Autodesk Inventor part; units mm, degrees
ref_plane "YZ Plane" through (0, 0, 0) normal (1, 0, 0) x (0, 1, 0)
ref_plane "XZ Plane" through (0, 0, 0) normal (0, 1, 0) x (-1, 0, 0)
ref_plane "XY Plane" through (0, 0, 0) normal (0, 0, 1) x (1, 0, 0)
sketch "スケッチ1" plane through (-150, -150, 0) normal (0, 0, 1) x (1, 0, 0)
  circle A0 centre (59.9853, 240.0147) radius 24 construction
  circle A1 centre (59.9853, 240.0147) radius 24 construction
  circle A2 centre (84.0269, 264.0563) radius 10 construction
  line L0 (84.0269, 264.0563) -> (59.9853, 240.0147) construction
  line L1 (59.9853, 240.0147) -> (84.0269, 215.9731) construction
  arc A3 (84.5273, 253.0677) -> (73.0383, 264.5567) centre (84.0269, 264.0563) ccw
  arc A4 (70.2215, 262.823) -> (82.7936, 250.2509) centre (59.9853, 240.0147) ccw
  arc A5 (84.5273, 253.0677) -> (82.7936, 250.2509) centre (84.6183, 251.0698) ccw
  arc A6 (70.2215, 262.823) -> (73.0383, 264.5567) centre (71.0404, 264.6477) ccw
  line L2 (67.0564, 275.37) -> (24.63, 232.9436) construction
  line L3 (24.63, 232.9436) -> (52.9142, 204.6594) construction
  line L4 (52.9142, 204.6594) -> (95.3406, 247.0858) construction
  line L5 (95.3406, 247.0858) -> (67.0564, 275.37) construction
  line L6 (67.0564, 275.37) -> (52.9142, 204.6594) construction
  line L7 (24.63, 232.9436) -> (95.3406, 247.0858) construction
  circle A7 centre (95.3406, 247.0858) radius 1.6
  circle A8 centre (52.9142, 204.6594) radius 1.6
  circle A9 centre (24.63, 232.9436) radius 1.6
  circle A10 centre (67.0564, 275.37) radius 1.6
  line L8 (270, 30) -> (30, 30) construction
  line L9 (30, 30) -> (30, 270) construction
  line L10 (30, 270) -> (270, 270) construction
  line L11 (270, 270) -> (270, 30) construction
  line L12 (270, 30) -> (30, 270) construction
  line L13 (30, 30) -> (270, 270) construction
  circle A11 centre (30, 270) radius 2 construction
  circle A12 centre (270, 270) radius 2 construction
  circle A13 centre (30, 30) radius 2
  circle A14 centre (270, 30) radius 2
  circle A15 centre (150, 150) radius 30
  line L14 (150, 113) -> (117.9571, 131.5) construction
  line L15 (117.9571, 131.5) -> (117.9571, 168.5) construction
  line L16 (117.9571, 168.5) -> (150, 187) construction
  line L17 (150, 187) -> (182.0429, 168.5) construction
  line L18 (182.0429, 168.5) -> (182.0429, 131.5) construction
  line L19 (182.0429, 131.5) -> (150, 113) construction
  circle A16 centre (150, 150) radius 37 construction
  circle A17 centre (150, 113) radius 1.6
  circle A18 centre (54.1207, 93.2509) radius 1.6 construction
  line L20 (117.9571, 131.5) -> (117.9571, 168.5) construction
  line L21 (150, 113) -> (117.9571, 131.5) construction
  line L22 (117.9571, 168.5) -> (150, 187) construction
  line L23 (182.0429, 131.5) -> (150, 113) construction
  circle A19 centre (150, 150) radius 30 construction
  line L24 (150, 187) -> (182.0429, 168.5) construction
  line L25 (182.0429, 168.5) -> (182.0429, 131.5) construction
  circle A20 centre (150, 150) radius 37 construction
  circle A21 centre (182.0429, 131.5) radius 1.6
  circle A22 centre (151.2065, 38.5916) radius 1.6 construction
  line L26 (150, 113) -> (117.9571, 131.5) construction
  line L27 (182.0429, 131.5) -> (150, 113) construction
  line L28 (117.9571, 131.5) -> (117.9571, 168.5) construction
  line L29 (182.0429, 168.5) -> (182.0429, 131.5) construction
  circle A23 centre (150, 150) radius 30 construction
  line L30 (117.9571, 168.5) -> (150, 187) construction
  line L31 (150, 187) -> (182.0429, 168.5) construction
  circle A24 centre (150, 150) radius 37 construction
  circle A25 centre (182.0429, 168.5) radius 1.6
  circle A26 centre (247.0858, 95.3406) radius 1.6 construction
  line L32 (182.0429, 131.5) -> (150, 113) construction
  line L33 (182.0429, 168.5) -> (182.0429, 131.5) construction
  line L34 (150, 113) -> (117.9571, 131.5) construction
  line L35 (150, 187) -> (182.0429, 168.5) construction
  circle A27 centre (150, 150) radius 30 construction
  line L36 (117.9571, 131.5) -> (117.9571, 168.5) construction
  line L37 (117.9571, 168.5) -> (150, 187) construction
  circle A28 centre (150, 150) radius 37 construction
  circle A29 centre (150, 187) radius 1.6
  circle A30 centre (245.8793, 206.7491) radius 1.6 construction
  line L38 (182.0429, 168.5) -> (182.0429, 131.5) construction
  line L39 (150, 187) -> (182.0429, 168.5) construction
  line L40 (182.0429, 131.5) -> (150, 113) construction
  line L41 (117.9571, 168.5) -> (150, 187) construction
  circle A31 centre (150, 150) radius 30 construction
  line L42 (150, 113) -> (117.9571, 131.5) construction
  line L43 (117.9571, 131.5) -> (117.9571, 168.5) construction
  circle A32 centre (150, 150) radius 37 construction
  circle A33 centre (117.9571, 168.5) radius 1.6
  circle A34 centre (148.7935, 261.4084) radius 1.6 construction
  line L44 (150, 187) -> (182.0429, 168.5) construction
  line L45 (117.9571, 168.5) -> (150, 187) construction
  line L46 (182.0429, 168.5) -> (182.0429, 131.5) construction
  line L47 (117.9571, 131.5) -> (117.9571, 168.5) construction
  circle A35 centre (150, 150) radius 30 construction
  line L48 (182.0429, 131.5) -> (150, 113) construction
  line L49 (150, 113) -> (117.9571, 131.5) construction
  circle A36 centre (150, 150) radius 37 construction
  circle A37 centre (117.9571, 131.5) radius 1.6
  line L50 (0, 300) -> (300, 300)
  line L51 (300, 300) -> (300, 0)
  line L52 (300, 0) -> (0, 0)
  line L53 (0, 0) -> (0, 300)
  line L54 (0, 300) -> (300, 0) construction
  line L55 (300, 300) -> (0, 0) construction
  point P0 (150, 150)
  point P1 (81.1985, 261.2279)
  point P2 (150, 150)
  point P3 (59.8791, 125.8522)
  point P4 (150, 150)
  point P5 (125.8522, 59.8791)
  point P6 (150, 150)
  point P7 (215.9731, 84.0269)
  point P8 (150, 150)
  point P9 (240.1209, 174.1478)
  point P10 (150, 150)
  point P11 (174.1478, 240.1209)
  dimension "d30" = 74
  dimension "d6" = 48
  dimension "d7" = 20
  dimension "d10" = 25
  dimension "d11" = 11
  dimension "d12" = 2
  dimension "d15" = 40
  dimension "d16" = 60
  dimension "d17" = 3.2
  dimension "d18" = 240
  dimension "d19" = 4
  dimension "d22" = 240
  dimension "d25" = 240
  dimension "d28" = 60
  dimension "d31" = 3.2
  dimension "d34" = 360
  dimension "d36" = 300
  dimension "d39" = 127.3
  dimension "d40" = 3.2
  dimension "d41" = 48
extrude "押し出し2" add sketch "スケッチ1" along normal blind 10
sketch "スケッチ2" plane through (-150, -150, 0) normal (0, 0, -1) x (-1, 0, 0)
  circle A0 centre (-150, 150) radius 90
  dimension "d42" = 180
extrude "押し出し3" cut sketch "スケッチ2" against normal blind 3
sketch "スケッチ3" plane through (-150, -150, 10) normal (0, 0, 1) x (1, 0, 0)
  line L0 (300, 300) -> (0, 300)
  line L1 (0, 300) -> (0, 0)
  line L2 (0, 0) -> (300, 0)
  line L3 (300, 0) -> (300, 300)
  circle A0 centre (150, 150) radius 30
  line L4 (150, 180) -> (150, 150) construction
  line L5 (50, 180) -> (50, 150)
  line L6 (250, 150) -> (250, 180)
  arc A1 (250, 180) -> (50, 180) centre (150, 180) ccw
  arc A2 (50, 150) -> (250, 150) centre (150, 150) ccw
  line L7 (50, 180) -> (0, 180)
  line L8 (250, 180) -> (300, 180)
  line L9 (300, 40) -> (0, 40)
  line L10 (64, 300) -> (34, 270)
  line L11 (266, 270) -> (236, 300)
  line L12 (300, 270) -> (266, 270)
  line L13 (34, 270) -> (0, 270)
  point P0 (150, 165)
  dimension "d45" = 100
  dimension "d46" = 30
  dimension "d51" = 40
  dimension "d52" = 45
  dimension "d53" = 64
  dimension "d55" = 30
extrude "押し出し5" cut sketch "スケッチ3" against normal blind 10 contours L3 L12 L11 L0 | L10 L13 L1 L0 | L3 L9 L1 L7 L5 A2 L6 L8 | L3 L2 L1 L9
sketch "スケッチ5" plane through (-150, -150, 10) normal (0, 0, 1) x (1, 0, 0)
  circle A0 centre (18, 187) radius 1.6
  circle A1 centre (282, 187) radius 1.6
  point P0 (150, 150)
  point P1 (18, 220)
  point P2 (282, 220)
  dimension "d65" = 33
  dimension "d66" = 33
hole "穴1" at (-132, 37, 10) at (132, 37, 10) at (132, 70, 10) at (-132, 70, 10) direction (0, 0, -1) diameter 3.2 end through all
fillet "フィレット1" radius 3 10 edges at (-86, 150, 5) (-116, 120, 5) (-150, 120, 5) (-150, 30, 5) (-100, 30, 5) (100, 30, 5) (150, 30, 5) (150, 120, 5) (116, 120, 5) (86, 150, 5)
properties part number "ロボットベース2019" material "マツ材"
Input: part model. Units: mm. Frame: model coordinates. A direction names the side the tool comes from. Give positions to 0.01 mm unless a question says otherwise; leave off trailing zeros. Write each loop counter-clockwise with the first axis right and the second up, starting at its lowest first coordinate (ties: lowest second). Pieces come first, ordered by that corner, then holes. Notation, with made-up numbers: M -3,22 L 36,22 A20 ccw 36,33 Z; hole C 12,-12 d4. An arc over 180 degrees is marked long. Use one line per item in the form item = value.
1. First-contact query: P1, Ø4, axis at x = -32.04, y = -18.5, coming from the -Z side; P2, Ø5, axis at x = -121.5, z = 6.5, coming from the -Y side; P3, Ø3, axis at x = -97.09, y = 54.66, coming from the +Z side; P4, Ø3, axis at x = 134, z = 5, coming from the +Y side. Flat tips, straight axial feed; report the tip coordinate or a pass-through.
Outcome:
P1 = 3
P2 = 30
P3 = through
P4 = 120
2. Cut plane A-A on y = -48. Return loops of the section in (x, z).
Outcome:
outline = M -87.73,0 L -76.13,0 L -76.13,3 L 76.13,3 L 76.13,0 L 87.73,0 L 87.73,10 L -87.73,10 Z
3. Cut plane C-C on z = 6. State how many separate pieces and enclosed holes the cut face has, and give its area (3 significant figures).
Outcome:
separate_pieces = 1
enclosed_holes = 16
area = 49,500 mm²
4. Mould query, pull axis X, two halves, no side actions, for faces 1 (the face through (-0.7, 90.4, 0)), 2 (the face through (-2.199, -99.976, 5.07)), 3 (the face through (-106.99, 71.66, 4.93)). Classes: released by +X, released by -X, zero draft, split by the parting line, or undercut.
Outcome:
face_1 = zero draft
face_2 = split by the parting line
face_3 = undercut
5. Ray query, L1, parallel to Y at x = -132, z = 7.5; L2, parallel to Y at x = 0, z = 8.25; L3, parallel to X at y = 37, z = 5.75. Return the intervals inside material, ascending.
Outcome:
L1 = 30 to 35.4, 38.6 to 68.4, 71.6 to 120
L2 = -100 to -38.6, -35.4 to -30, 30 to 35.4, 38.6 to 150
L3 = -150 to -133.6, -130.4 to -1.6, 1.6 to 130.4, 133.6 to 150
6. Cut plane B-B on x = 122.5. Return loops of the section in (y, z).
Outcome:
outline = M 30,0 L 120,0 L 120,10 L 30,10 Z
7. Reachability of faces 4 (the face through (-132, 120, 5)), 5 (the face through (-125, 30, 5)), 6 (the face through (132, 120, 5)), 7 (the face through (125, 30, 5)), 8 (the face through (-41.53, -79.845, 1.479)) from +Z, -Z, +X, -X, +Y, -Y: full face, straight path, thin tool, end or side. Return the list, or none.
Outcome:
face_4 = +Z, -Z, -X, +Y
face_5 = +Z, -Z, -X, -Y
face_6 = +Z, -Z, +X, +Y
face_7 = +Z, -Z, +X, -Y
face_8 = -Z
8. Cut plane D-D on x = 51. Return loops of the section in (y, z).
Outcome:
outline = M -86.02,0 L -74.16,0 L -74.16,3 L 74.16,3 L 74.16,0 L 150,0 L 150,10 L -86.02,10 Z
